The listing builds one solid part. Answer for the finished solid, in the listing's coordinates (mm). Give positions to 0.01 mm unless a question says otherwise; leave off trailing zeros. Order: outer loops, then holes, each group sorted by start corner. A loop starts at its lowest first (then second) coordinate and runs counter-clockwise, first axis right, second up. Notation, with made-up numbers: (78.5, 37) - (128.5, 37) arc R14 ccw to (128.5, 45) - close; hole circle Ø11 at (-10, 42). An arc over 180 degrees is marked (long way). Answer as CSV lines item,"result". Start each with the question number.
1. Section A-A on x = -0.2 is taken. Give the vertices of the cut face in (y, z), and give its area (3 significant figures).
2. Section B-B on y = 1.25 is taken. Give the vertices of the cut face in (x, z).
3. Section C-C on z = -10 is taken. Give the vertices of the cut face in (x, y).
4. Flat-ended cylindrical pins translate along their axes: pin 1 (1 mm diameter, centred on y = 4.5, z = -7.5, fed in from -X); pin 2 (1.5 mm diameter, centred on x = 1.5, z = -12, fed in from -Y); pin 3 (3.5 mm diameter, centred on y = 2.5, z = -4, fed in from +X). Find the tip coordinate at first contact, or state that the pin passes through.
5. Consider line 1 along X through (y, z) = (2.75, -2.75); line 2 along Z through (x, y) = (-1.5, 1); line 3 along Y through (x, z) = (-1, -6.25). Determine where each line is inside the solid, lowest interval first. Write a range as [from, to].
from build123d import *

# Parameters (mm, degrees)
SKETCH1_R                = 0.3
BOSS_EXTRUDE1_DEPTH      = 2.5
BOSS_EXTRUDE2_DEPTH      = 2
BOSS_EXTRUDE2_DEPTH_BACK = 2


with BuildPart() as part:
    # Sketch1 → Boss-Extrude1 (new, symmetric)
    with BuildSketch(Plane(origin=(0, 0, 0), x_dir=(0, 0, -1), z_dir=(1, 0, 0))):
        Circle(SKETCH1_R)
    extrude(amount=BOSS_EXTRUDE1_DEPTH, both=True)

    # Sketch2 → Boss-Extrude2 (add, two sides: drawn at the far end of the back side and taken through both)
    with BuildSketch(Plane(origin=(0, 0, 0), x_dir=(0, 0, -1), z_dir=(1, 0, 0)).offset(-BOSS_EXTRUDE2_DEPTH_BACK)):
        with BuildLine():
            Line((-0.296211166, 0.047528362), (-0.296211166, 2.047528362))
            ThreePointArc((-0.296211166, 2.047528362), (-0.233869415, 2.231181239), (-0.07260959, 2.338931609))
            Line((-0.07260959, 2.338931609), (15.7, 6.565189611))
            Line((15.7, 6.565189611), (15.853330182, 5.992953581))
            Line((15.853330182, 5.992953581), (0.296211166, 1.824436104))
            Line((0.296211166, 1.824436104), (0.296211166, 0.047528362))
            Line((0.296211166, 0.047528362), (-0.296211166, 0.047528362))
        make_face()
    extrude(amount=BOSS_EXTRUDE2_DEPTH + BOSS_EXTRUDE2_DEPTH_BACK)


solid = part.part
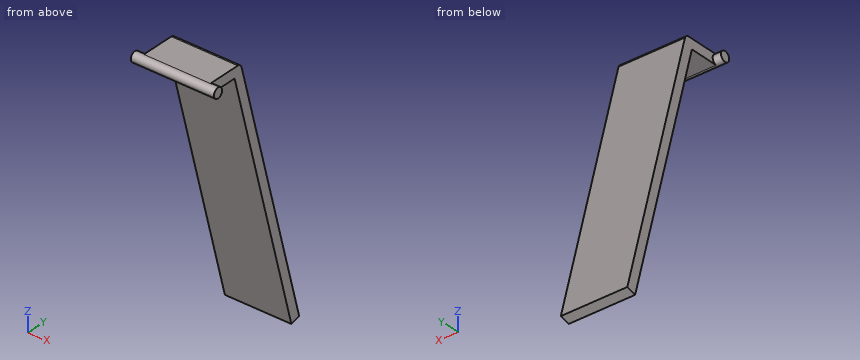
Checks:
1,outline,"(0.05, -0.3) - (1.82, -0.3) - (5.99, -15.85) - (6.57, -15.7) - (2.34, 0.07) arc R0.3 ccw to (2.05, 0.3) - (0.05, 0.3) arc R0.3 ccw (long way) to start"
1,area,"11.0 mm²"
2,outline,"(-2, -0.3) - (2, -0.3) - (2, 0.3) - (-2, 0.3) - close"
3,outline,"(-2, 4.42) - (2, 4.42) - (2, 5.04) - (-2, 5.04) - close"
4,pin 1,"stops at x = -2"
4,pin 2,"stops at y = 4.76"
4,pin 3,"stops at x = 2"
5,line 1,"x = [-2, 2]"
5,line 2,"z = [-0.3, 0.3]"
5,line 3,"y = [3.42, 4.03]"
